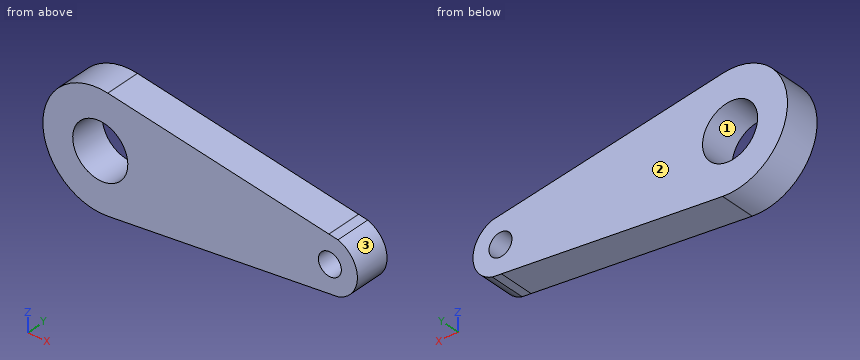
from build123d import *

# Parameters (mm, degrees)
SKETCH1_R           = 152.4
SKETCH1_R_2         = 63.5
BOSS_EXTRUDE1_DEPTH = 190.5


with BuildPart() as part:
    # Sketch1 → Boss-Extrude1 (new body)
    with BuildSketch(Plane(origin=(0, 0, 0), x_dir=(1, 0, 0), z_dir=(0, 1, 0))):
        with BuildLine():
            Line((657.371733042, 152.307316196), (-565.509397264, 314.735802206))
            ThreePointArc((-565.509397264, 314.735802206), (-924.814, 0), (-565.509397264, -314.735802206))
            Line((-565.509397264, -314.735802206), (657.371733042, -152.307316196))
            Line((657.371733042, -152.307316196), (707.57483155, -145.639118379))
            ThreePointArc((707.57483155, -145.639118379), (815.086, 0), (707.57483155, 145.639118379))
            Line((707.57483155, 145.639118379), (657.371733042, 152.307316196))
        make_face()
        with Locations(Location((-607.314, 0, 0), (0, 0, 270))):
            Circle(SKETCH1_R, mode=Mode.SUBTRACT)
        with Locations(Location((662.686, 0, 0), (0, 0, 270))):
            Circle(SKETCH1_R_2, mode=Mode.SUBTRACT)
    extrude(amount=BOSS_EXTRUDE1_DEPTH)


solid = part.part
Could you check a few things on this model? Use its own coordinates, in mm. Face numbers are marked on the shaded views. Give positions to 0.01 mm unless a question says otherwise; leave off trailing zeros. Order: outer loops, then holes, each group sorted by start corner. A loop starts at its lowest first (then second) coordinate and runs counter-clockwise, first axis right, second up. Notation, with made-up numbers: (71, 23.5) - (112, 23.5) arc R13 cw to (112, 27.5) - close; hole circle Ø10 at (19.25, 39). An arc over 180 degrees is marked (long way). One line per item, written item: value. Start each with the question number.
1. For P1, Ø1.5, axis at x = 357.5, y = 53.5, coming from the +Z side; P2, Ø6, axis at y = 147, z = 45, coming from the -X side; P3, Ø1, axis at x = -678, y = 42.5, coming from the +Z side, each with a flat end and sliding along its axis, tell me the tip position at first contact or that it passes through.
2. Thinking about a two-plate mould opening in Z: for the marked faces 1, 2 and 3, which applies, +Z half, -Z half, draft (parallel to the pull), parting line (faces both ways), or undercut?
3. Imagine slicing it at D-D on z = 252.5. List the corners of the cut face in (x, y) for me.
4. Imagine slicing it at B-B on x = -534.5. List the corners of the cut face in (y, z) for me.
5. Imagine slicing it at C-C on y = 133. List the corners of the cut face in (x, z) for me.
6. If I drill on probe 1 along X at (y, z) = (135.5, -11); probe 2 along X at (y, z) = (122, 46); probe 3 along X at (y, z) = (47.5, 108), over which ranges is the centre line in solid material (lowest first)?
7. Imagine slicing it at A-A on z = 0. List the corners of the cut face in (x, y) for me.
Values:
1. P1: z = 192.24
1. P2: x = -922.02
1. P3: z = 309.65
2. face 1: undercut
2. face 2: draft
2. face 3: parting line
3. outline: (-799.8, 0) - (-96.95, 0) - (-96.95, 190.5) - (-799.8, 190.5) - close
4. outline: (0, -310.62) - (190.5, -310.62) - (190.5, -133.88) - (0, -133.88) - close; (0, 133.88) - (190.5, 133.88) - (190.5, 310.62) - (0, 310.62) - close
5. outline: (-565.51, -314.74) - (707.57, -145.64) arc R152.4 ccw to (707.57, 145.64) - (-565.51, 314.74) arc R317.5 ccw (long way) to start; hole circle Ø304.8 at (-607.31, 0); hole circle Ø127 at (662.69, 0)
6. probe 1: -924.62 to -759.32, -455.31 to 600.15, 725.23 to 814.69
6. probe 2: -921.46 to -752.61, -462.02 to 618.91, 706.46 to 807.98
6. probe 3: -905.88 to -714.84, -499.79 to 770.21
7. outline: (-924.81, 0) - (-759.71, 0) - (-759.71, 190.5) - (-924.81, 190.5) - close; (-454.91, 0) - (599.19, 0) - (599.19, 190.5) - (-454.91, 190.5) - close; (726.19, 0) - (815.09, 0) - (815.09, 190.5) - (726.19, 190.5) - close
